Can you work these out from the model? Positions are in its coordinate system, mm. Give positions to 0.01 mm unless a question says otherwise; leave off trailing zeros. Write each loop counter-clockwise with the first axis right and the second up, starting at its lowest first coordinate (ties: lowest second). Pieces come first, ordered by that corner, then holes.
from build123d import *

# Parameters (mm, degrees)
SKETCH2_W           = 780
SKETCH2_H           = 380
BOSS_EXTRUDE1_DEPTH = 2
SKETCH3_W           = 30
SKETCH3_H           = 30
CUT_EXTRUDE1_DEPTH  = 3
SKETCH4_R           = 3.25
CUT_EXTRUDE2_DEPTH  = 3
SKETCH5_R           = 7.5
CUT_EXTRUDE3_DEPTH  = 3
CUT_EXTRUDE4_DEPTH  = 3


with BuildPart() as part:
    # Sketch2 → Boss-Extrude1 (new body)
    with BuildSketch(Plane(origin=(0, 0, 0), x_dir=(1, 0, 0), z_dir=(0, 1, 0))):
        Rectangle(SKETCH2_W, SKETCH2_H)
    extrude(amount=BOSS_EXTRUDE1_DEPTH)

    # Sketch3 → Cut-Extrude1 (cut, through all)
    with BuildSketch(Plane(origin=(0, 2, 0), x_dir=(1, 0, 0), z_dir=(0, 1, 0))):
        with Locations((-375, 175)):
            Rectangle(SKETCH3_W, SKETCH3_H)
        with Locations((375, 175)):
            Rectangle(SKETCH3_W, SKETCH3_H)
        with Locations((375, -175)):
            Rectangle(SKETCH3_W, SKETCH3_H)
        with Locations((-375, -175)):
            Rectangle(SKETCH3_W, SKETCH3_H)
    extrude(amount=-CUT_EXTRUDE1_DEPTH, mode=Mode.SUBTRACT)

    # Sketch4 → Cut-Extrude2 (cut, through all)
    with BuildSketch(Plane(origin=(0, 2, 0), x_dir=(1, 0, 0), z_dir=(0, 1, 0))):
        with Locations((-375, 0)):
            Circle(SKETCH4_R)
        with Locations((375, 0)):
            Circle(SKETCH4_R)
        with Locations((-160, 175)):
            Circle(SKETCH4_R)
        with Locations((160, 175)):
            Circle(SKETCH4_R)
        with Locations((-160, -175)):
            Circle(SKETCH4_R)
        with Locations((160, -175)):
            Circle(SKETCH4_R)
    extrude(amount=-CUT_EXTRUDE2_DEPTH, mode=Mode.SUBTRACT)

    # Sketch5 → Cut-Extrude3 (cut, through all)
    with BuildSketch(Plane(origin=(0, 2, 0), x_dir=(1, 0, 0), z_dir=(0, 1, 0))):
        with Locations((-220, -16)):
            Circle(SKETCH5_R)
    extrude(amount=-CUT_EXTRUDE3_DEPTH, mode=Mode.SUBTRACT)

    # Sketch6 → Cut-Extrude4 (cut, through all)
    with BuildSketch(Plane(origin=(0, 2, 0), x_dir=(1, 0, 0), z_dir=(0, 1, 0))):
        with BuildLine():
            Line((-32, 75), (162, 75))
            ThreePointArc((162, 75), (164.121320344, 74.121320344), (165, 72))
            Line((165, 72), (165, 23))
            ThreePointArc((165, 23), (164.121320344, 20.878679656), (162, 20))
            Line((162, 20), (-32, 20))
            ThreePointArc((-32, 20), (-34.121320344, 20.878679656), (-35, 23))
            Line((-35, 23), (-35, 72))
            ThreePointArc((-35, 72), (-34.121320344, 74.121320344), (-32, 75))
        make_face()
    extrude(amount=-CUT_EXTRUDE4_DEPTH, mode=Mode.SUBTRACT)


solid = part.part
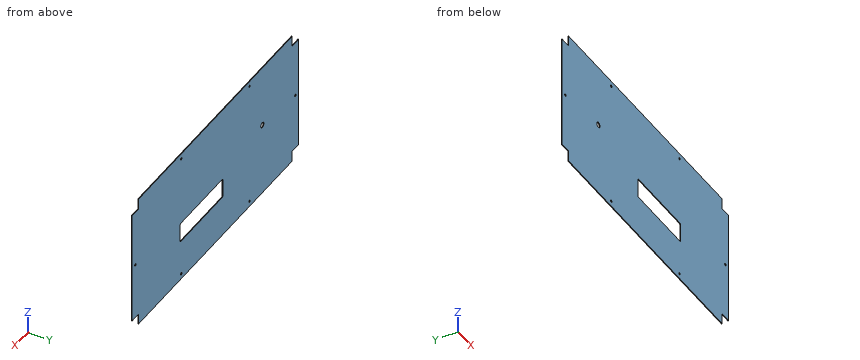
(1) Imagine slicing it at B-B, the plane z = 16. Write out the boundary of the cut face in (x, y).
Returned:
outline: (-390, 0) - (-227.5, 0) - (-227.5, 2) - (-390, 2) - close; (-212.5, 0) - (390, 0) - (390, 2) - (-212.5, 2) - close
(2) Will these pins go through, and if not, where does the flat tip stop? P1, Ø6, axis at x = 160, z = -175, coming from the +Y side; P2, Ø0.6, axis at x = -368, y = 0.5, coming from the -Z side; P3, Ø0.6, axis at y = 1, z = -181, coming from the -X side; P4, Ø0.6, axis at x = 370.5, y = 1.5, coming from the +Z side.
Returned:
P1: passes through
P2: stops at z = -160
P3: stops at x = -360
P4: stops at z = 160
(3) Imagine slicing it at A-A, the plane x = 46. Write out the boundary of the cut face in (y, z), plus the area to 3 significant figures.
Returned:
outline: (0, -190) - (2, -190) - (2, -75) - (0, -75) - close; (0, -20) - (2, -20) - (2, 190) - (0, 190) - close
area: 650 mm2
(4) If I drill on L1, parallel to Z at x = -160, y = 1.45; L2, parallel to Z at x = 160, y = 1; L3, parallel to X at y = 0.85, z = 175, over which ranges is the centre line in solid material (lowest first)?
Returned:
L1: z = -190 to -178.25, -171.75 to 171.75, 178.25 to 190
L2: z = -190 to -178.25, -171.75 to -75, -20 to 171.75, 178.25 to 190
L3: x = -360 to -163.25, -156.75 to 156.75, 163.25 to 360
(5) Imagine slicing it at C-C, the plane y = 1.25. Give the number of separate pieces and of enclosed holes in the cut face, plus the area to 3 significant figures.
Returned:
separate pieces: 1
enclosed holes: 8
area: 281,000 mm2
